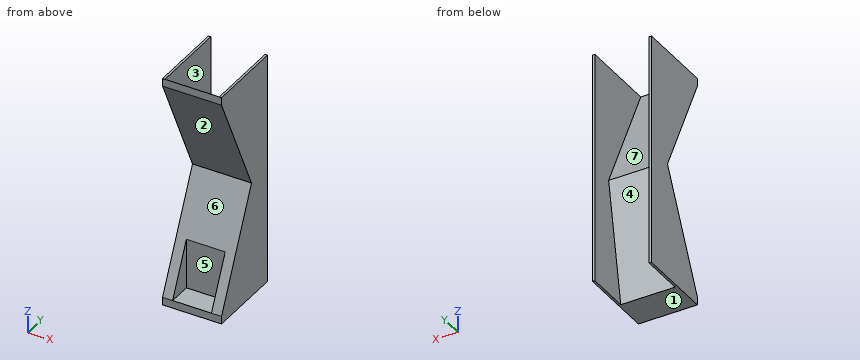
```python
from build123d import *

# Parameters (mm, degrees)
SKETCH1_W           = 70
SKETCH1_H           = 300
BOSS_EXTRUDE1_DEPTH = 70
SKETCH1_4_W         = 3
SKETCH1_4_H         = 300
BOSS_EXTRUDE2_DEPTH = 100
CUT_EXTRUDE1_DEPTH  = 70
CUT_EXTRUDE2_DEPTH  = 70
CUT_EXTRUDE3_DEPTH  = 205.769718293
SKETCH10_W          = 50
SKETCH10_H          = 70
CUT_EXTRUDE4_DEPTH  = 30


with BuildPart() as part:
    # Sketch1 → Boss-Extrude1 (new body)
    with BuildSketch(Plane(origin=(0, 0, 0), x_dir=(1, 0, 0), z_dir=(0, 1, 0))):
        with Locations((-11.73177624, -11.723954719)):
            Rectangle(SKETCH1_W, SKETCH1_H)
    extrude(amount=BOSS_EXTRUDE1_DEPTH)

    # Sketch1<4> → Boss-Extrude2 (add)
    with BuildSketch(Plane(origin=(0, 0, 0), x_dir=(1, 0, 0), z_dir=(0, 1, 0))):
        with Locations((-48.23177624, -11.723954719)):
            Rectangle(SKETCH1_4_W, SKETCH1_4_H)
        with Locations((24.76822376, -11.723954719)):
            Rectangle(SKETCH1_4_W, SKETCH1_4_H)
    extrude(amount=BOSS_EXTRUDE2_DEPTH)

    # Sketch2 → Cut-Extrude1 (cut)
    with BuildSketch(Plane.ZY.offset(46.73177624)):
        Polygon((161.723954719, 70), (11.608470283, 70), (161.723954719, 0), align=None)
    extrude(amount=-CUT_EXTRUDE1_DEPTH, mode=Mode.SUBTRACT)

    # Sketch3 → Cut-Extrude2 (cut)
    with BuildSketch(Plane.ZY.offset(46.73177624)):
        Polygon((11.608470283, 70), (-138.276045281, 70), (-138.276045281, 43.571315916), align=None)
    extrude(amount=-CUT_EXTRUDE2_DEPTH, mode=Mode.SUBTRACT)

    # Sketch8 → Cut-Extrude3 (cut, through all)
    with BuildSketch(Plane(origin=(26.26822376, 0, 0), x_dir=(0, 0, -1), z_dir=(1, 0, 0))):
        Polygon((-151.723954719, 0), (-11.723954719, 65.283072142), (128.276045281, 0), (-11.723954719, 0), align=None)
    extrude(amount=-CUT_EXTRUDE3_DEPTH, mode=Mode.SUBTRACT)

    # Sketch10 → Cut-Extrude4 (cut)
    with BuildSketch(Plane.XZ):
        with Locations((-11.73177624, -93.276045281)):
            Rectangle(SKETCH10_W, SKETCH10_H)
    extrude(amount=-CUT_EXTRUDE4_DEPTH, mode=Mode.SUBTRACT)


solid = part.part
```
The model under review builds one solid part; all positions refer to its coordinate system, in mm. Face numbers are marked on the shaded views. A direction names the side the tool comes from. Give positions to 0.01 mm unless a question says otherwise; leave off trailing zeros. Write each loop counter-clockwise with the first axis right and the second up, starting at its lowest first coordinate (ties: lowest second). Pieces come first, ordered by that corner, then holes. Notation, with made-up numbers: (8, 3) - (42, 3) arc R19 cw to (42, 20) - close; hole circle Ø8 at (-3, 85.5). An arc over 180 degrees is marked (long way). Answer in a Markdown table with one row per item. Add a question column.
1. We need section C-C on z = -112. Write out the cut boundary in (x, y).
2. Draft analysis for pull direction Z (two halves, no side actions). For the marked faces 1, 2 and 3, state which applies: +Z half, -Z half, draft (parallel to the pull), parting line (faces both ways), or undercut.
3. Wall thickness on line 1 along X through (y, z) = (56, 96); line 2 along X through (y, z) = (26, -82.5); line 3 along Z through (x, y) = (-30, 10.5): over which ranges is each line inside the solid? List them lowest first. Write a range as [from, to].
4. We need section B-B on x = -1.5. Write out the cut boundary in (y, z), then the cut area to 3 significant figures.
5. We need section D-D on y = 24.5. Write out the cut boundary in (x, z), then the cut area to 3 significant figures.
6. Tool access review of the marked faces 4, 5, 6 and 7: name each direction out of +Z, -Z, +X, -X, +Y, -Y from which nothing blocks a thin tool from reaching the whole face with its end or side.
7. We need section A-A on y = 73. Write out the cut boundary in (x, z).
8. Insertion check: P1, Ø5, axis at x = -35, y = 30, coming from the +Z side; P2, Ø24, axis at x = -2, y = 21.5, coming from the +Z side; P3, Ø1, axis at x = -23, y = 27.5, coming from the +Z side. Each pin has a flat end and moves straight along its axis. Give the tip position at first contact, or say it passes through.
Ans:
| question | item | result |
|---|---|---|
| 1 | outline | (-49.73, 7.59) - (-36.73, 7.59) - (-36.73, 30) - (13.27, 30) - (13.27, 7.59) - (26.27, 7.59) - (26.27, 100) - (23.27, 100) - (23.27, 48.2) - (-46.73, 48.2) - (-46.73, 100) - (-49.73, 100) - close |
| 2 | face 1 | -Z half |
| 2 | face 2 | undercut |
| 2 | face 3 | draft |
| 3 | line 1 | x = [-49.73, -46.73], [23.27, 26.27] |
| 3 | line 2 | x = [-49.73, -36.73], [13.27, 26.27] |
| 3 | line 3 | z = [-138.28, -128.28], [129.21, 139.21] |
| 4 | outline | (0, -138.28) - (43.57, -138.28) - (70, 11.61) - (0, 161.72) - (0, 151.72) - (65.28, 11.72) - (30, -63.94) - (30, -128.28) - (0, -128.28) - close |
| 4 | area | 3,660 mm^2 |
| 5 | outline | (-49.73, -138.28) - (26.27, -138.28) - (26.27, -75.74) - (13.27, -75.74) - (13.27, -128.28) - (-36.73, -128.28) - (-36.73, -75.74) - (-49.73, -75.74) - close; (-49.73, 99.18) - (26.27, 99.18) - (26.27, 161.72) - (23.27, 161.72) - (23.27, 109.18) - (-46.73, 109.18) - (-46.73, 161.72) - (-49.73, 161.72) - close |
| 5 | area | 3,200 mm^2 |
| 6 | face 4 | -Z, +Y |
| 6 | face 5 | -Y |
| 6 | face 6 | +X, -X, -Y |
| 6 | face 7 | +Z, +Y |
| 7 | outline | (-49.73, -138.28) - (-46.73, -138.28) - (-46.73, 161.72) - (-49.73, 161.72) - close; (23.27, -138.28) - (26.27, -138.28) - (26.27, 161.72) - (23.27, 161.72) - close |
| 8 | P1 | stops at z = 102.75 |
| 8 | P2 | stops at z = 141.35 |
| 8 | P3 | stops at z = 103.82 |
